```python
from build123d import *

# Parameters (mm, degrees)
F1_DEPTH = 25
F2_T     = 2
F4_W     = 10.5
F4_H     = 4
F5_DEPTH = 3


# Not quite as in the source:
# - a shell that OpenCascade refuses in one call is made with other operations: the cavity is built on its own and cut out


with BuildPart() as f1:
    # F0 (on Top) → F1 (new body)
    with BuildSketch(Plane.XY):
        with BuildLine():
            Line((24, 16), (-24, 16))
            ThreePointArc((-24, 16), (-25.4142135624, 15.4142135624), (-26, 14))
            Line((-26, 14), (-26, -14))
            ThreePointArc((-26, -14), (-25.4142135624, -15.4142135624), (-24, -16))
            Line((-24, -16), (24, -16))
            ThreePointArc((24, -16), (25.4142135624, -15.4142135624), (26, -14))
            Line((26, -14), (26, 14))
            ThreePointArc((26, 14), (25.4142135624, 15.4142135624), (24, 16))
        make_face()
    extrude(amount=F1_DEPTH)

    # F2: shell of thickness 2, made by hand


with BuildPart() as f2_core1:
    # F2_t2: copy of F1
    add(f1.part)

    # the walls: a layer under each face that stays
    f2_faces = [f2_core1.faces().sort_by_distance(p)[0] for p in [
        (0, 16, 12.5),
        (-26, 0, 12.5),
        (0, -16, 12.5),
        (26, 0, 12.5),
        (0, 0, 0),
    ]]
    thicken(f2_faces, amount=-F2_T, mode=Mode.SUBTRACT)


with BuildPart() as f1_1:
    add(f1.part)

    # what is left inside the walls is the cavity
    f2_cavity = [f2_core1.part.solids().sort_by_distance(p)[0] for p in [
        (0, -4.666667, 2.02),
    ]]
    add(f2_cavity, mode=Mode.SUBTRACT)

    # F4 (on offset) → F5 (cut)
    with BuildSketch(Plane.YZ.offset(25.5)):
        with Locations((0, 4)):
            Rectangle(F4_W, F4_H)
    extrude(amount=-F5_DEPTH, mode=Mode.SUBTRACT)


solid = f1_1.part
```
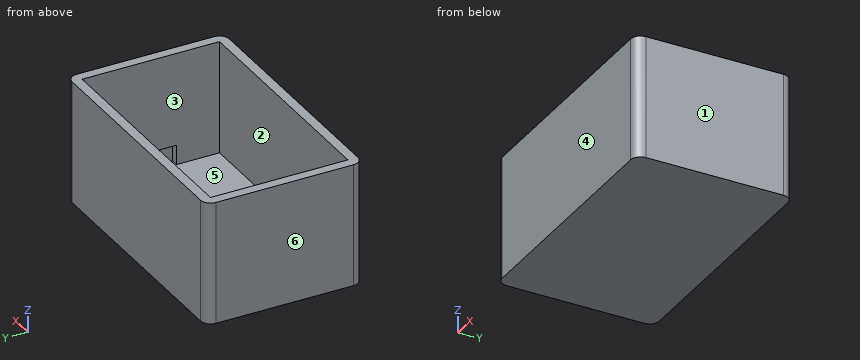
Here's how the part is built. I have some questions about the finished solid (model axes, mm). Face numbers are marked on the shaded views. A direction names the side the tool comes from. Coordinates: 2 decimals unless noted, no trailing zeros. Write each loop counter-clockwise with the first axis right and the second up, starting at its lowest first coordinate (ties: lowest second). Pieces come first, ordered by that corner, then holes. Notation, with made-up numbers: (-18, 63) -> (-7, 63) arc R20 cw to (-7, 89) -> close; hole circle Ø2 at (44.5, 22). An arc over 180 degrees is marked (long way). Use a Markdown table: item, result. Add a question column.
(1) If we section it at D-D, the plane z = 4.5: Write out the boundary of the cut face in (x, y).
(2) If we section it at C-C, the plane y = -1: Write out the boundary of the cut face in (x, z), and give its area (3 significant figures).
(3) Please list where these lines run through material, in increasing order: line 1 (X direction, y = -6, z = 10.25); line 2 (Y direction, x = 20, z = 22.25); line 3 (Z direction, x = 3, y = 7.5).
(4) If we section it at B-B, the plane x = -8: Write out the boundary of the cut face in (y, z), and give its area (3 significant figures).
(5) If we section it at A-A, the plane z = 17.25: Write out the boundary of the cut face in (x, y), and give its area (3 significant figures).
(6) I'm going to push a flat-ended pin straight in: P1, Ø1, axis at x = -2.5, y = -3, coming from the +Z side. Where does the tip first touch, or does it pass through?
(7) We'd pull the mould along Y, two halves only. Please class the marked faces 3, 4, 5 and 6: +Y half, -Y half, draft (parallel to the pull), parting line (faces both ways), or undercut.
(8) For the marked faces 1 and 2, which set-ups out of +Z, -Z, +X, -X, +Y, -Y let a thin tool reach every point of the face, with its end or its side?
Outcome:
| question | item | result |
|---|---|---|
| 1 | outline | (-26, -14) arc R2 ccw to (-24, -16) -> (24, -16) arc R2 ccw to (26, -14) -> (26, 14) arc R2 ccw to (24, 16) -> (-24, 16) arc R2 ccw to (-26, 14) -> close; hole (-24, -14) -> (24, -14) -> (24, -5.25) -> (25.5, -5.25) -> (25.5, 5.25) -> (24, 5.25) -> (24, 14) -> (-24, 14) -> close |
| 2 | outline | (-26, 0) -> (26, 0) -> (26, 25) -> (24, 25) -> (24, 6) -> (25.5, 6) -> (25.5, 2) -> (-24, 2) -> (-24, 25) -> (-26, 25) -> close |
| 2 | area | 190 mm^2 |
| 3 | line 1 | x = -26 to -24, 24 to 26 |
| 3 | line 2 | y = -16 to -14, 14 to 16 |
| 3 | line 3 | z = 0 to 2 |
| 4 | outline | (-16, 0) -> (16, 0) -> (16, 25) -> (14, 25) -> (14, 2) -> (-14, 2) -> (-14, 25) -> (-16, 25) -> close |
| 4 | area | 156 mm^2 |
| 5 | outline | (-26, -14) arc R2 ccw to (-24, -16) -> (24, -16) arc R2 ccw to (26, -14) -> (26, 14) arc R2 ccw to (24, 16) -> (-24, 16) arc R2 ccw to (-26, 14) -> close; hole (-24, -14) -> (24, -14) -> (24, 14) -> (-24, 14) -> close |
| 5 | area | 317 mm^2 |
| 6 | P1 | stops at z = 2 |
| 7 | face 3 | undercut |
| 7 | face 4 | -Y half |
| 7 | face 5 | undercut |
| 7 | face 6 | draft |
| 8 | face 1 | +Z, -Z, +X, +Y, -Y |
| 8 | face 2 | +Z |
